Work out the finished part from the listing and answer in its coordinate system (mm). Face numbers are marked on the shaded views. A direction names the side the tool comes from. Coordinates: 2 decimals unless noted, no trailing zeros. Loops run counter-clockwise (first coordinate to the right, second up) from the corner with the lowest first, then second, coordinate; pieces in that order, holes last. Notation, with made-up numbers: M 24.5,-27 L 71.5,-27 A27 ccw 71.5,-2 Z; hole C 74.25,25 d4. An arc over 180 degrees is marked long. Write each question's results on one line, items separated by ' | '.
```python
from build123d import *

# Parameters (mm, degrees)
SKETCH5_W           = 50.8
SKETCH5_H           = 25.4
BOSS_EXTRUDE4_DEPTH = 1.5875
FILLET1_R           = 1.5875
SKETCH6_R           = 1.27
CUT_EXTRUDE1_DEPTH  = 29.442400677
SKETCH7_R           = 7.9375
BOSS_EXTRUDE5_DEPTH = 12.7
SKETCH8_R           = 6.35
CUT_EXTRUDE2_DEPTH  = 0.79375
FILLET2_R           = 0.396875
SKETCH9_W           = 10.16
SKETCH9_H           = 7.9375
BOSS_EXTRUDE6_DEPTH = 5.08
SKETCH10_R          = 0.426470585
SKETCH10_R_2        = 0.479624958
SKETCH10_R_3        = 0.577856792
SKETCH10_R_4        = 0.481547326
SKETCH10_W          = 3.81
SKETCH10_H          = 10.16
SKETCH10_W_2        = 8.89
SKETCH10_H_2        = 3.81
BOSS_EXTRUDE7_DEPTH = 1.5875


with BuildPart() as part:
    # Sketch5 → Boss-Extrude4 (new body)
    with BuildSketch(Plane(origin=(0, 0, 0), x_dir=(1, 0, 0), z_dir=(0, 1, 0))):
        Rectangle(SKETCH5_W, SKETCH5_H)
    extrude(amount=-BOSS_EXTRUDE4_DEPTH)

    # Fillet1
    fillet1_edges = [part.edges().sort_by_distance(p)[0] for p in [
        (25.4, -0.79375, 12.7),
        (-25.4, -0.79375, 12.7),
        (-25.4, -0.79375, -12.7),
        (25.4, -0.79375, -12.7),
    ]]
    fillet(fillet1_edges, radius=FILLET1_R)

    # Sketch6 → Cut-Extrude1 (cut, through all)
    with BuildSketch(Plane(origin=(0, 0, 0), x_dir=(1, 0, 0), z_dir=(0, 1, 0))):
        with Locations(Location((-22.86, 0, 0), (0, 0, 270))):
            Circle(SKETCH6_R)
        with Locations(Location((6.35, 10.16, 0), (0, 0, 270))):
            Circle(SKETCH6_R)
        with Locations(Location((6.35, -10.16, 0), (0, 0, 270))):
            Circle(SKETCH6_R)
    extrude(amount=-CUT_EXTRUDE1_DEPTH, mode=Mode.SUBTRACT)

    # Sketch7 → Boss-Extrude5 (add)
    with BuildSketch(Plane(origin=(0, 0, 0), x_dir=(1, 0, 0), z_dir=(0, 1, 0))):
        with Locations(Location((11.1125, 0, 0), (0, 0, 90))):
            Circle(SKETCH7_R)
        with Locations(Location((-11.1125, 0, 0), (0, 0, 90))):
            Circle(SKETCH7_R)
    extrude(amount=BOSS_EXTRUDE5_DEPTH)

    # Sketch8 → Cut-Extrude2 (cut)
    with BuildSketch(Plane(origin=(0, 12.7, 0), x_dir=(1, 0, 0), z_dir=(0, 1, 0))):
        with Locations(Location((-11.1125, 0, 0), (0, 0, 270))):
            Circle(SKETCH8_R)
        with Locations(Location((11.1125, 0, 0), (0, 0, 270))):
            Circle(SKETCH8_R)
    extrude(amount=-CUT_EXTRUDE2_DEPTH, mode=Mode.SUBTRACT)

    # Fillet2
    fillet2_edges = [part.edges().sort_by_distance(p)[0] for p in [
        (11.1125, 12.7, 7.9375),
        (-11.1125, 12.7, 7.9375),
        (-11.1125, 12.7, -6.35),
        (11.1125, 12.7, -6.35),
    ]]
    fillet(fillet2_edges, radius=FILLET2_R)

    # Sketch9 → Boss-Extrude6 (add)
    with BuildSketch(Plane(origin=(0, 0, 0), x_dir=(1, 0, 0), z_dir=(0, 1, 0))):
        with Locations((0, -10.31875)):
            Rectangle(SKETCH9_W, SKETCH9_H)
    extrude(amount=BOSS_EXTRUDE6_DEPTH)

    # Sketch10 → Boss-Extrude7 (add)
    with BuildSketch(Plane.XZ.offset(1.5875)):
        with Locations(Location((-11.075588504, 7.114058657, 0), (0, 0, 270))):
            Circle(SKETCH10_R)
        with Locations(Location((-11.1125, -7.019355369, 0), (0, 0, 270))):
            Circle(SKETCH10_R_2)
        with Locations(Location((11.3645169, -7.019355369, 0), (0, 0, 270))):
            Circle(SKETCH10_R_3)
        with Locations(Location((11.3645169, 7.114058657, 0), (0, 0, 270))):
            Circle(SKETCH10_R_4)
        with Locations((-17.362669173, 0)):
            Rectangle(SKETCH10_W, SKETCH10_H)
        with Locations((16.820766285, 0)):
            Rectangle(SKETCH10_W_2, SKETCH10_H_2)
        with Locations((-3.443063383, -4.515309272)):
            Rectangle(SKETCH10_W_2, SKETCH10_H_2)
    extrude(amount=BOSS_EXTRUDE7_DEPTH)


solid = part.part
```
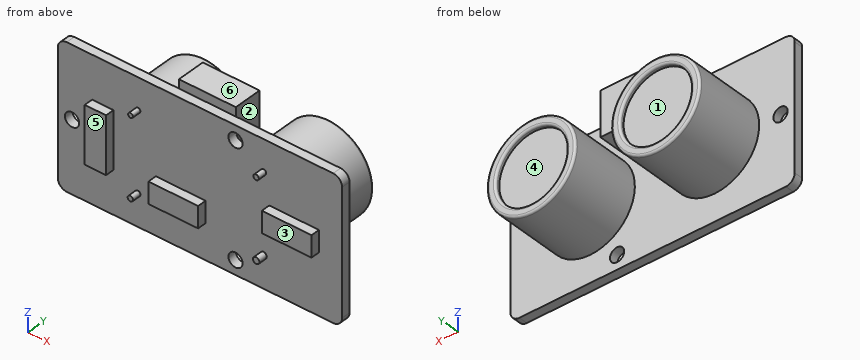
1) For a pull along Z with two mould halves and no side action, classify the marked faces 4, 5 and 6 as released by +Z, released by -Z, zero draft, split by the parting line, or undercut.
Check result:
face 4: undercut | face 5: zero draft | face 6: released by +Z
2) Which of the six approach directions +Z, -Z, +X, -X, +Y, -Y give full straight-line access (tool end or side, diameter ignored) to the marked faces 1, 2 and 3?
Check result:
face 1: +Y | face 2: +Z, +Y | face 3: +Z, -Z, +X, -X, -Y
3) Find section B-B, the plane x = -22.86. Give the vertices of the cut face in (y, z), and give its area (3 significant figures).
Check result:
outline: M -1.59,-12.7 L 0,-12.7 L 0,-1.27 L -1.59,-1.27 Z; M -1.59,1.27 L 0,1.27 L 0,12.7 L -1.59,12.7 Z | area: 36.3 mm^2
4) Given pin 1 Ø1 at (x, z) = (13, 6) entering from -Y; pin 2 Ø5.5 at (x, y) = (-1.5, 3.5) entering from -Z; pin 3 Ø1.3 at (y, z) = (-2.5, -2) entering from +X, each flat-ended and moving along its own axis, determine where each tip first touches the part or whether it passes through.
Check result:
pin 1: y = -1.59 | pin 2: z = -3.99 | pin 3: x = 21.27
5) Find section C-C, the plane y = 0.5. Give the number of separate pieces and of enclosed holes in the cut face, and give its area (3 significant figures).
Check result:
separate pieces: 3 | enclosed holes: 0 | area: 477 mm^2
6) Find section A-A, the plane z = -10.16. Give the vertices of the cut face in (x, y), and give its area (3 significant figures).
Check result:
outline: M -25.4,-1.59 L 5.08,-1.59 L 5.08,0 L -25.4,0 Z; M 7.62,-1.59 L 25.4,-1.59 L 25.4,0 L 7.62,0 Z | area: 76.6 mm^2
7) Find section D-D, the plane y = 10.75. Give the vertices of the cut face in (x, z) (1 decimal), and give its area (3 significant figures).
Check result:
outline: C -11.1,0 d15.9; C 11.1,0 d15.9 | area: 396 mm^2
8) Straight lines are drawn through the part: probe 1 along X at (y, z) = (-1.75, 0.25); probe 2 along X at (y, z) = (-0.55, 0); probe 3 along Y at (x, z) = (-11, -6.25). For each, find the intervals that lie inside material, in ascending order. Write a range as [from, to].
Check result:
probe 1: [-19.27, -15.46], [12.38, 21.27] | probe 2: [-25.4, -24.13], [-21.59, 25.4] | probe 3: [-1.59, 11.91]
